```python
from build123d import *

# Parameters (mm, degrees)
F0_R     = 10
F1_DEPTH = 40
F2_R     = 3.4
F3_DEPTH = 40.001
F4_W     = 25.61774
F4_H     = 10
F5_DEPTH = 2


with BuildPart() as f1:
    # F0 (on Top) → F1 (new body)
    with BuildSketch(Plane.XY):
        Circle(F0_R)
    extrude(amount=-F1_DEPTH)

    # F2 (on face) → F3 (cut, through all)
    with BuildSketch(Plane.XY):
        Circle(F2_R)
    extrude(amount=-F3_DEPTH, mode=Mode.SUBTRACT)

    # F4 (on face) → F5 (cut)
    with BuildSketch(Plane.XY):
        Rectangle(F4_W, F4_H)
    extrude(amount=-F5_DEPTH, mode=Mode.SUBTRACT)


solid = f1.part
```
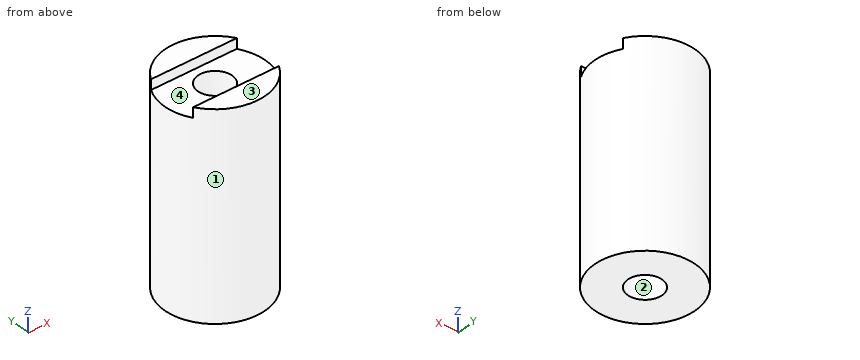
Work out the finished part from the listing and answer in its coordinate system (mm). Face numbers are marked on the shaded views. Coordinates: 2 decimals unless noted, no trailing zeros. Order: outer loops, then holes, each group sorted by start corner. A loop starts at its lowest first (then second) coordinate and runs counter-clockwise, first axis right, second up. Notation, with made-up numbers: (16.5, 66) - (34.5, 66) arc R28 cw to (34.5, 94) - close; hole circle Ø4 at (-35, 16.5). An arc over 180 degrees is marked (long way). Answer as a JSON object with one key per item and string values.
1. Find section C-C on z = -26.5. Determine the outline of the cut face in (x, y).
Output values:
{"outline": "circle Ø20 at (0, 0); hole circle Ø6.8 at (0, 0)"}
2. Find section B-B on y = 0. Determine the outline of the cut face in (x, z), plus the area to 3 significant figures.
Output values:
{"outline": "(-10, -40) - (-3.4, -40) - (-3.4, -2) - (-10, -2) - close; (3.4, -40) - (10, -40) - (10, -2) - (3.4, -2) - close", "area": "502 mm²"}
3. Find section A-A on x = 0. Determine the outline of the cut face in (y, z).
Output values:
{"outline": "(-10, -40) - (-3.4, -40) - (-3.4, -2) - (-5, -2) - (-5, 0) - (-10, 0) - close; (3.4, -40) - (10, -40) - (10, 0) - (5, 0) - (5, -2) - (3.4, -2) - close"}
4. Find section D-D on x = 8.25. Determine the outline of the cut face in (y, z).
Output values:
{"outline": "(-5.65, -40) - (5.65, -40) - (5.65, 0) - (5, 0) - (5, -2) - (-5, -2) - (-5, 0) - (-5.65, 0) - close"}
5. Each of these flat-tipped pins is pushed along its axis until it touches: P1, Ø2, axis at x = 3, z = -0.5, coming from the -Y side; P2, Ø1, axis at x = -4.5, z = -27, coming from the -Y side; P3, Ø2, axis at x = -2, z = -0.5, coming from the +Y side. Where does it stop, or does it pass through?
Output values:
{"P1": "stops at y = -9.8", "P2": "stops at y = -9.17", "P3": "stops at y = 9.95"}
6. The mould has two halves that part along Y. Classify the marked faces 1, 2, 3 and 4: +Y half, -Y half, draft (parallel to the pull), parting line (faces both ways), or undercut.
Output values:
{"face 1": "parting line", "face 2": "undercut", "face 3": "draft", "face 4": "undercut"}
7. Consider line 1 (Y direction, x = 0, z = -10.5); line 2 (Z direction, x = -6.5, y = -2.75); line 3 (X direction, y = 0.5, z = -26). Determine where each line is inside the solid, lowest interval first.
Output values:
{"line 1": "y = -10 to -3.4, 3.4 to 10", "line 2": "z = -40 to -2", "line 3": "x = -9.99 to -3.36, 3.36 to 9.99"}
